Build history of the part. All positions in model axes, mm. A direction names the side the tool comes from. Coordinates: 2 decimals unless noted, no trailing zeros. Loops run counter-clockwise (first coordinate to the right, second up) from the corner with the lowest first, then second, coordinate; pieces in that order, holes last.
(1) Slice it at A-A (y = 0). Give the cut face in (x, z).
(2) Flat gauge pins, fed straight in: P1, Ø1.3, axis at x = -44, z = 0.5, coming from the +Y side; P2, Ø8, axis at y = 3.5, z = 7, coming from the +X side; P3, Ø0.7, axis at x = -46, y = 7.5, coming from the +Z side. Where does each tip first touch, or does it go through?
(3) Wall check: L1, parallel to X at y = -3.75, z = 0; L2, parallel to X at y = -5, z = 0; L3, parallel to X at y = 5, z = -4.5. Give the ranges that are in metal, low to high.
(4) Slice it at B-B (x = 25). Give the cut face in (y, z), and give its area (3 significant figures).
(5) Slice it at D-D (z = -7). Give the cut face in (x, y), and give its area (3 significant figures).
(6) Two-plate mould, pull along X, no slides. Class faces 4 (the face through (-5.07, -4.55, -1.5)), 5 (the face through (-56.941, -0.867, 3.905)), 6 (the face through (-54, 2, 4)): pulls with the +X half, pulls with the -X half, needs draft (parallel to the pull), parting line crosses it, or undercut.
(7) Tool access for faces 1 (the face through (0, -8, 0)), 2 (the face through (0, -1, 0)), 3 (the face through (-35, 6, -6)): list every direction of +Z, -Z, +X, -X, +Y, -Y with a clear straight run to the whole face (end or side of a thin tool).
(8) Slice it at C-C (y = -5.5). Give the cut face in (x, z).
Autodesk Inventor part; units mm, degrees
ref_plane "YZ Plane" through (0, 0, 0) normal (1, 0, 0) x (0, 1, 0)
ref_plane "XZ Plane" through (0, 0, 0) normal (0, 1, 0) x (-1, 0, 0)
ref_plane "XY Plane" through (0, 0, 0) normal (0, 0, 1) x (1, 0, 0)
sketch "Esboço1" plane through (0, 0, 0) normal (0, 0, 1) x (1, 0, 0)
  line L0 (-30, 8) -> (28.9137, 8)
  line L1 (28.9137, 0) -> (28.9137, 8)
  line L2 (-30, 8) -> (-30, 14)
  line L3 (-30, 14) -> (-35, 14)
  line L4 (-35, 14) -> (-35, 8)
  line L5 (-35, 8) -> (-54, 8)
  line L6 (-54, 8) -> (-54, 4)
  line L7 (-54, 4) -> (-60, 4)
  line L8 (-60, 4) -> (-60, 0)
  line L9 (-60, 0) -> (28.9137, 0)
  point P0 (0, 0)
  dimension "d2" = 6
  dimension "d3" = 5
  dimension "d4" = 6
  dimension "d5" = 19
  dimension "d6" = 4
  dimension "d7" = 6
revolve "Revolução1" add sketch "Esboço1" angle 360 about axis through (-60, 0, 0) along (1, 0, 0)
sketch "Esboço2" plane through (0, 0, 0) normal (0, 1, 0) x (-1, 0, 0)
  line L0 (-28.9137, 8) -> (-28.9137, -8)
  line L1 (30, 8) -> (30, -8)
  line L2 (-28.9137, 8) -> (30, 8)
  line L3 (30, 8) -> (30, -8)
  line L4 (30, -8) -> (-28.9137, -8)
  line L5 (-28.9137, -8) -> (-28.9137, 8)
  point P0 (0, 0)
extrude "Extrusão1" cut sketch "Esboço2" along normal blind 10 and the other way blind 1
sketch "Esboço3" plane through (0, -1, 0) normal (0, 1, 0) x (1, 0, 0)
  line L0 (-30, -14) -> (-30, 14)
  point P0 (0, 0)
  point P1 (-5, 0)
  point P2 (25, 0)
  dimension "d13" = 25
  dimension "d14" = 30
hole "Furo1" at (-5, -1, 0) at (25, -1, 0) direction (0, -1, 0) diameter 3 end through all
thread "Rosca1"
fillet "Arredondamento1" radius 0.2 1 edges at (-60, -4, 0)
sketch "Esboço4" plane through (-54, 0, 0) normal (-1, 0, 0) x (0, 0, 1)
  circle A0 centre (0, 0) radius 8
  line L0 (0, 8) -> (0.6, 8)
  line L1 (0.6, 8) -> (0.6, 6.6)
  line L2 (0.6, 6.6) -> (0, 6.6)
  line L3 (0, 6.6) -> (0, 8)
  line L4 (0, 8) -> (-0.6, 8)
  line L5 (-0.6, 8) -> (-0.6, 6.6)
  line L6 (-0.6, 6.6) -> (0, 6.6)
  line L7 (0, 6.6) -> (0, 8)
  point P0 (0.6, 7.9775)
  point P1 (-0.6, 7.9775)
  dimension "d25" = 0.6
  dimension "d26" = 1.4
  dimension "d27" = 0.6
  dimension "d28" = 1.4
extrude "Extrusão2" cut sketch "Esboço4" against normal blind 14 contours L1 L2 L3 A0 | A0 L3 L6 L5
properties part number "Eixo"
Response values:
1. outline: (-60, -3.8) arc R0.2 ccw to (-59.8, -4) - (-54, -4) - (-54, -8) - (-35, -8) - (-35, -14) - (-30, -14) - (-30, 14) - (-35, 14) - (-35, 8) - (-54, 8) - (-54, 4) - (-59.8, 4) arc R0.2 ccw to (-60, 3.8) - close
2. P1: stops at y = 7.98
2. P2: stops at x = -30
2. P3: stops at z = 3.59
3. L1: x = -60 to -6.5, -3.5 to 23.5, 26.5 to 28.91
3. L2: x = -54 to -6.5, -3.5 to 23.5, 26.5 to 28.91
3. L3: x = -54 to -30
4. outline: (-7.86, -1.5) arc R8 ccw to (-1, -7.94) - (-1, -1.5) - close; (-7.86, 1.5) - (-1, 1.5) - (-1, 7.94) arc R8 ccw to start
4. area: 63.7 mm2
5. outline: (-54, -3.87) - (-35, -3.87) - (-35, -12.12) - (-30, -12.12) - (-30, -3.87) - (28.91, -3.87) - (28.91, -1) - (-30, -1) - (-30, 12.12) - (-35, 12.12) - (-35, 3.87) - (-54, 3.87) - close
5. area: 438 mm2
6. face 4: undercut
6. face 5: needs draft
6. face 6: pulls with the -X half
7. face 1: +X, -Y
7. face 2: +Z, -Z, +X, +Y
7. face 3: -X
8. outline: (-54, -5.81) - (-35, -5.81) - (-35, -12.87) - (-30, -12.87) - (-30, -5.81) - (28.91, -5.81) - (28.91, 5.81) - (-30, 5.81) - (-30, 12.87) - (-35, 12.87) - (-35, 5.81) - (-54, 5.81) - close; hole circle Ø3 at (-5, 0); hole circle Ø3 at (25, 0)
